from build123d import *

# Parameters (mm, degrees)
SKETCH1_R           = 5.08
SKETCH1_R_2         = 0.3175
BOSS_EXTRUDE1_DEPTH = 1.5875
CUT_EXTRUDE1_DEPTH  = 8.357510194
FILLET1_R           = 0.508
FILLET2_R           = 0.508


with BuildPart() as part:
    # Sketch1 → Boss-Extrude1 (new body)
    with BuildSketch(Plane(origin=(0, 0, 0), x_dir=(1, 0, 0), z_dir=(0, 1, 0))):
        with Locations(Location((0, 0, 0), (0, 0, 270))):
            Circle(SKETCH1_R)
        with Locations(Location((0, 0, 0), (0, 0, 270))):
            Circle(SKETCH1_R_2, mode=Mode.SUBTRACT)
    extrude(amount=BOSS_EXTRUDE1_DEPTH)

    # Sketch2 → Cut-Extrude1 (cut, through all)
    with BuildSketch(Plane(origin=(0, 1.5875, 0), x_dir=(1, 0, 0), z_dir=(0, 1, 0))):
        with BuildLine():
            Line((-0.71842049, 0.71842049), (-0.71842049, 3.76642049))
            ThreePointArc((-0.71842049, 3.76642049), (-2.873681959, 2.873681959), (-3.76642049, 0.71842049))
            Line((-3.76642049, 0.71842049), (-0.71842049, 0.71842049))
        make_face()
        with BuildLine():
            Line((0.71842049, 0.71842049), (3.76642049, 0.71842049))
            ThreePointArc((3.76642049, 0.71842049), (2.873681959, 2.873681959), (0.71842049, 3.76642049))
            Line((0.71842049, 3.76642049), (0.71842049, 0.71842049))
        make_face()
        with BuildLine():
            Line((0.71842049, -0.71842049), (3.76642049, -0.71842049))
            ThreePointArc((3.76642049, -0.71842049), (2.873681959, -2.873681959), (0.71842049, -3.76642049))
            Line((0.71842049, -3.76642049), (0.71842049, -0.71842049))
        make_face()
        with BuildLine():
            Line((-0.71842049, -0.71842049), (-0.71842049, -3.76642049))
            ThreePointArc((-0.71842049, -3.76642049), (-2.873681959, -2.873681959), (-3.76642049, -0.71842049))
            Line((-3.76642049, -0.71842049), (-0.71842049, -0.71842049))
        make_face()
    extrude(amount=-CUT_EXTRUDE1_DEPTH, mode=Mode.SUBTRACT)

    # Fillet1
    fillet1_edges = [part.edges().sort_by_distance(p)[0] for p in [
        (-0.71842049, 0.79375, -0.71842049),
        (0.71842049, 0.79375, -0.71842049),
        (0.71842049, 0.79375, 0.71842049),
        (-0.71842049, 0.79375, 0.71842049),
    ]]
    fillet(fillet1_edges, radius=FILLET1_R)

    # Fillet2
    fillet2_edges = [part.edges().sort_by_distance(p)[0] for p in [
        (-3.76642049, 0.79375, -0.71842049),
        (-0.71842049, 0.79375, -3.76642049),
        (0.71842049, 0.79375, -3.76642049),
        (3.76642049, 0.79375, -0.71842049),
        (0.71842049, 0.79375, 3.76642049),
        (3.76642049, 0.79375, 0.71842049),
        (-3.76642049, 0.79375, 0.71842049),
        (-0.71842049, 0.79375, 3.76642049),
    ]]
    fillet(fillet2_edges, radius=FILLET2_R)


solid = part.part
Design review of the part built by this model. Coordinates are the model's own, in mm. A direction names the side the tool comes from. Round coordinates to 2 decimals unless told otherwise and drop trailing zeros. Write each loop counter-clockwise with the first axis right and the second up, starting at its lowest first coordinate (ties: lowest second). Pieces come first, ordered by that corner, then holes.
Item 1: For pin 1 Ø1.5 at (x, z) = (3.5, -1.5) entering from +Y; pin 2 Ø0.5 at (y, z) = (0.5, 2) entering from +X; pin 3 Ø0.8 at (x, y) = (-2.5, 0.5) entering from +Z; pin 4 Ø0.5 at (y, z) = (0.5, -2.5) entering from -X, all flat-tipped, find the tip position at first contact; note any pin that passes through.
Item 2: Consider section D-D on x = -1.5. Give the boundary of the cut face in (y, z), and give its area (3 significant figures).
Item 3: Consider section B-B on z = 0. Give the boundary of the cut face in (x, y).
Item 4: Wall thickness on L1, parallel to X at y = 1.1, z = 0; L2, parallel to X at y = 0.55, z = -2.25; L3, parallel to X at y = 1.5, z = -2.5: over which ranges is each line inside the solid? List them lowest first.
Item 5: Consider section C-C on y = 1. Give the boundary of the cut face in (x, z) (1 decimal), and give its area (3 significant figures).
Item 6: Draft analysis for pull direction X (two halves, no side actions). For faces 3 (the flat face through (2, 1, -0.718)), 4 (the cylindrical face through (5.037, 0.783, -0.661)), 5 (the flat face through (-1, 1.588, 0)), state which applies: released by +X, released by -X, zero draft, split by the parting line, or undercut.
Item 7: Consider section A-A on x = 0. Give the boundary of the cut face in (y, z).
Item 8: For faces 1 (the flat face through (-2, 1, 0.718)), 2 (the flat face through (-1, 0, 0)), list the 3-axis set-ups (+Z, -Z, +X, -X, +Y, -Y) from which the entire face can be reached by the end or side of a thin tool; tool diameter is ignored.
Check values:
1. pin 1: stops at y = 1.59
1. pin 2: stops at x = 4.77
1. pin 3: stops at z = 4.63
1. pin 4: stops at x = -4.55
2. outline: (0, -4.85) - (1.59, -4.85) - (1.59, -3.66) - (0, -3.66) - close; (0, -0.72) - (1.59, -0.72) - (1.59, 0.72) - (0, 0.72) - close; (0, 3.66) - (1.59, 3.66) - (1.59, 4.85) - (0, 4.85) - close
2. area: 6.06 mm2
3. outline: (-5.08, 0) - (-0.32, 0) - (-0.32, 1.59) - (-5.08, 1.59) - close; (0.32, 0) - (5.08, 0) - (5.08, 1.59) - (0.32, 1.59) - close
4. L1: x = -5.08 to -0.32, 0.32 to 5.08
4. L2: x = -4.55 to -3.35, -0.72 to 0.72, 3.35 to 4.55
4. L3: x = -4.42 to -3.19, -0.72 to 0.72, 3.19 to 4.42
5. outline: circle Ø10.2 at (0, 0); hole (-3.7, -1.3) arc R3 ccw to (-1.3, -3.7) arc R0.5 ccw to (-0.7, -3.2) - (-0.7, -1.2) arc R0.5 ccw to (-1.2, -0.7) - (-3.2, -0.7) arc R0.5 ccw to start; hole (-3.7, 1.3) arc R0.5 ccw to (-3.2, 0.7) - (-1.2, 0.7) arc R0.5 ccw to (-0.7, 1.2) - (-0.7, 3.2) arc R0.5 ccw to (-1.3, 3.7) arc R3 ccw to start; hole circle Ø0.6 at (0, 0); hole (0.7, -3.2) arc R0.5 ccw to (1.3, -3.7) arc R3 ccw to (3.7, -1.3) arc R0.5 ccw to (3.2, -0.7) - (1.2, -0.7) arc R0.5 ccw to (0.7, -1.2) - close; hole (0.7, 1.2) arc R0.5 ccw to (1.2, 0.7) - (3.2, 0.7) arc R0.5 ccw to (3.7, 1.3) arc R3 ccw to (1.3, 3.7) arc R0.5 ccw to (0.7, 3.2) - close
5. area: 52.4 mm2
6. face 3: undercut
6. face 4: split by the parting line
6. face 5: zero draft
7. outline: (0, -5.08) - (1.59, -5.08) - (1.59, -0.32) - (0, -0.32) - close; (0, 0.32) - (1.59, 0.32) - (1.59, 5.08) - (0, 5.08) - close
8. face 1: +Y, -Y
8. face 2: +Z, -Z, +X, -X, -Y
